from build123d import *

# Parameters (mm, degrees)
ESQUISSE1_W                     = 45
ESQUISSE1_H                     = 23
EXTRUSION1_DEPTH                = 13.4
ENL_V_MAT_EXTRU_1_DEPTH         = 29.601748198
ENL_V_MAT_EXTRU_1_DEPTH_BACK    = 29.601748198
ENL_V_MAT_EXTRU_2_DEPTH         = 29.601748198
ENL_V_MAT_EXTRU_2_DEPTH_BACK    = 29.601748198
CONG_1_R                        = 3
ENL_V_MAT_EXTRU_3_DEPTH         = 29.601748198
ENL_V_MAT_EXTRU_3_DEPTH_BACK    = 29.601748198
ESQUISSE5_W                     = 8.2
ESQUISSE5_H                     = 18.2
ENL_V_MAT_EXTRU_4_DEPTH         = 6.75
ESQUISSE6_R                     = 1.5
EXTRUSION2_DEPTH                = 2
ESQUISSE7_R                     = 0.55
EXTRUSION3_DEPTH                = 20
EXTRUSION4_REACH                = 49.875
ESQUISSE8_W                     = 0.65
ESQUISSE8_H                     = 0.65
R_P_TITION_LIN_AIRE1_COUNT      = 3
R_P_TITION_LIN_AIRE1_PITCH      = 2.5
R_P_TITION_LIN_AIRE1_COUNT_DIR2 = 7
R_P_TITION_LIN_AIRE1_PITCH_DIR2 = 2.5
EXTRUSION5_DEPTH                = 0.2
R_P_TITION_LIN_AIRE2_COUNT      = 7
R_P_TITION_LIN_AIRE2_PITCH      = 2.5


with BuildPart() as part:
    # Esquisse1 → Extrusion1 (new body)
    with BuildSketch(Plane(origin=(0, 0, 0), x_dir=(1, 0, 0), z_dir=(0, 1, 0))):
        Rectangle(ESQUISSE1_W, ESQUISSE1_H)
    extrude(amount=EXTRUSION1_DEPTH)

    # Esquisse2 → Enlèv. mat.-Extru.1 (cut, two sides: drawn at the far end of the back side and taken through both)
    with BuildSketch(Plane.XY.offset(-ENL_V_MAT_EXTRU_1_DEPTH_BACK)):
        Polygon((22.5, 13.4), (22.5, 9), (-6.807961623, 9), (-10.5, 13.4), align=None)
    extrude(amount=ENL_V_MAT_EXTRU_1_DEPTH + ENL_V_MAT_EXTRU_1_DEPTH_BACK, mode=Mode.SUBTRACT)

    # Esquisse3 → Enlèv. mat.-Extru.2 (cut, two sides: drawn at the far end of the back side and taken through both)
    with BuildSketch(Plane(origin=(0, 0, 0), x_dir=(0, 0, -1), z_dir=(1, 0, 0)).offset(-ENL_V_MAT_EXTRU_2_DEPTH_BACK)):
        Polygon((18.471230279, -53.558334344), (11.5, 5), (10.5, 13.4), (-10.5, 13.4), (-11.5, 5), (-18.471230279, -53.558334344), (-18.471230279, 64.385322929), (18.471230279, 64.385322929), align=None)
    extrude(amount=ENL_V_MAT_EXTRU_2_DEPTH + ENL_V_MAT_EXTRU_2_DEPTH_BACK, mode=Mode.SUBTRACT)

    # Congé1
    cong_1_edges = [part.edges().sort_by_distance(p)[0] for p in [
        (22.5, 9, 0),
    ]]
    fillet(cong_1_edges, radius=CONG_1_R)

    # Esquisse4 → Enlèv. mat.-Extru.3 (cut, two sides: drawn at the far end of the back side and taken through both)
    with BuildSketch(Plane(origin=(0, 0, 0), x_dir=(1, 0, 0), z_dir=(0, 1, 0)).offset(-ENL_V_MAT_EXTRU_3_DEPTH_BACK)):
        Polygon((133.574230148, 11.5), (22.5, 11.5), (19, 11.5), (42, 0), (19, -11.5), (22.5, -11.5), (133.574230148, -11.5), (355.722690444, -11.5), (355.722690444, 11.5), align=None)
    extrude(amount=ENL_V_MAT_EXTRU_3_DEPTH + ENL_V_MAT_EXTRU_3_DEPTH_BACK, mode=Mode.SUBTRACT)

    # Esquisse5 → Enlèv. mat.-Extru.4 (cut)
    with BuildSketch(Plane(origin=(0, 13.4, 0), x_dir=(-1, 0, 0), z_dir=(0, 1, 0))):
        with Locations((16.5, 0)):
            Rectangle(ESQUISSE5_W, ESQUISSE5_H)
    extrude(amount=-ENL_V_MAT_EXTRU_4_DEPTH, mode=Mode.SUBTRACT)

    # Esquisse6 → Extrusion2 (add)
    with BuildSketch(Plane(origin=(22.5, 0, 0), x_dir=(0, 0, -1), z_dir=(1, 0, 0))):
        with Locations(Location((0, 2.5, 0), (0, 0, 180))):
            Circle(ESQUISSE6_R)
    extrude(amount=EXTRUSION2_DEPTH)

    # Esquisse7 → Extrusion3 (add)
    with BuildSketch(Plane(origin=(24.5, 0, 0), x_dir=(0, 0, -1), z_dir=(1, 0, 0))):
        with Locations((0, 2.5)):
            Circle(ESQUISSE7_R)
    extrude(amount=EXTRUSION3_DEPTH)

    # Esquisse8 → Extrusion4 (add, up to next)
    with BuildSketch(Plane(origin=(0, 13.4, 0), x_dir=(-1, 0, 0), z_dir=(0, 1, 0)), mode=Mode.PRIVATE) as extrusion4_sk1:
        with Locations((14, -7.5)):
            Rectangle(ESQUISSE8_W, ESQUISSE8_H)
    extrusion4_tool1 = extrude(extrusion4_sk1.sketch, amount=-EXTRUSION4_REACH, mode=Mode.PRIVATE) - part.part
    extrusion4 = extrusion4_tool1.solids().sort_by_distance((-14, 13.4, -7.5))[0]
    add(extrusion4)

    # Répétition linéaire1: Extrusion4 3 × 7
    with Locations(*[(-i * R_P_TITION_LIN_AIRE1_PITCH, 0, j * R_P_TITION_LIN_AIRE1_PITCH_DIR2) for i in range(R_P_TITION_LIN_AIRE1_COUNT) for j in range(R_P_TITION_LIN_AIRE1_COUNT_DIR2) if (i, j) != (0, 0)]):
        add(extrusion4)

    # Esquisse9 → Extrusion5 (add)
    with BuildSketch(Plane(origin=(0.436559012, 0.366316506, 0), x_dir=(0, 0, -1), z_dir=(0.766044443118982, 0.6427876096865347, 0))):
        with BuildLine():
            Line((7.175, 12.467369403), (7.175, 15.817369403))
            ThreePointArc((7.175, 15.817369403), (7.5, 16.142369403), (7.825, 15.817369403))
            Line((7.825, 15.817369403), (7.825, 12.467369403))
            ThreePointArc((7.825, 12.467369403), (7.5, 12.142369403), (7.175, 12.467369403))
        make_face()
    extrusion5 = extrude(amount=EXTRUSION5_DEPTH)

    # Répétition linéaire2: Extrusion5 ×7
    with Locations(*[(0, 0, i * R_P_TITION_LIN_AIRE2_PITCH) for i in range(1, R_P_TITION_LIN_AIRE2_COUNT)]):
        add(extrusion5)


solid = part.part
Here's how the part is built. I have some questions about the finished solid (model axes, mm). A direction names the side the tool comes from. Coordinates: 2 decimals unless noted, no trailing zeros. Write each loop counter-clockwise with the first axis right and the second up, starting at its lowest first coordinate (ties: lowest second). Pieces come first, ordered by that corner, then holes.
1) If I drill on line 1 (X direction, y = 6.25, z = 4.5); line 2 (Z direction, x = -17, y = 9.25); line 3 (X direction, y = 7, z = 7.75) (3 decimals), over which ranges is the centre line in solid material (lowest first)?
Filled in:
line 1: x = -22.5 to 22.49
line 2: z = -10.99 to -9.1, 9.1 to 10.99
line 3: x = -22.5 to -20.6, -19.325 to -18.675, -16.825 to -16.175, -14.325 to -13.675, -12.4 to 22.328
2) If we section it at D-D (x = -15): List the corners of the cut face in (y, z) for me.
Filled in:
outline: (0, -11.5) - (5, -11.5) - (13.4, -10.5) - (13.4, -9.1) - (6.65, -9.1) - (6.65, 9.1) - (13.4, 9.1) - (13.4, 10.5) - (5, 11.5) - (0, 11.5) - close
3) Which directions (+Z, -Z, +X, -X, +Y, -Y) give clear straight access to the entire face, cutting with the end or side of a thin tool? Please do faces 4 (the face through (20.726, 4.421, -10.637)), 5 (the face through (-12.4, 10, 0)).
Filled in:
face 4: -Z, +X, +Y, -Y
face 5: +Y
4) I'm going to push flat-ended pins straight in: pin 1 (0.5 mm diameter, centred on x = -19, y = 11, fed in from -Z); pin 2 (1 mm diameter, centred on x = 9.5, y = 11, fed in from +Z); pin 3 (0.5 mm diameter, centred on x = -19, y = 9.5, fed in from +Z); pin 4 (0.5 mm diameter, centred on x = -14, y = 8.5, fed in from +Z). Where does each tip first touch, or does it pass through?
Filled in:
pin 1: stops at z = -10.82
pin 2: passes through
pin 3: stops at z = 10.99
pin 4: stops at z = 11.11
5) If we section it at A-A (z = -6): List the corners of the cut face in (x, y) for me.
Filled in:
outline: (-22.5, 0) - (22.5, 0) - (22.5, 6) arc R3 ccw to (19.5, 9) - (-6.81, 9) - (-10.5, 13.4) - (-12.4, 13.4) - (-12.4, 6.65) - (-20.6, 6.65) - (-20.6, 13.4) - (-22.5, 13.4) - close
6) If we section it at C-C (y = 8): Count the separate pieces of the cut face and the enclosed holes in it, plus the area to 3 significant figures.
Filled in:
separate pieces: 22
enclosed holes: 1
area: 843 mm2
7) If we section it at B-B (x = 6): List the corners of the cut face in (y, z) for me.
Filled in:
outline: (0, -11.5) - (5, -11.5) - (9, -11.02) - (9, 11.02) - (5, 11.5) - (0, 11.5) - close
8) Thinking about a two-plate mould opening in Z: for faces 1 (the face through (-22.5, 7, 0)), 2 (the face through (34.36, 2.96, -0.3)), 3 (the face through (-16, 10, 9.1)), which applies, +Z half, -Z half, draft (parallel to the pull), parting line (faces both ways), or undercut?
Filled in:
face 1: draft
face 2: parting line
face 3: undercut
